from build123d import *

# Parameters (mm, degrees)
SKETCH1_R                = 10
BOSS_EXTRUDE1_DEPTH      = 50
EXTRUDE_THIN1_START      = -15
SKETCH2_R                = 11
SKETCH2_R_2              = 10
EXTRUDE_THIN1_DEPTH      = 15
SKETCH3_R                = 5
BOSS_EXTRUDE2_DEPTH      = 66
CUT_EXTRUDE3_DEPTH       = 118.038455219
CUT_EXTRUDE3_DEPTH_BACK  = 118.038455219
SKETCH4_R                = 2
EXTRUDE_THIN2_DEPTH      = 12
EXTRUDE_THIN2_DEPTH_BACK = 12
SKETCH5_R                = 11
SKETCH5_R_2              = 10
CUT_EXTRUDE4_DEPTH       = 118.038455318
CUT_EXTRUDE4_DEPTH_BACK  = 118.038455318
SKETCH7_R                = 2


with BuildPart() as part:
    # Sketch1 → Boss-Extrude1 (new body)
    with BuildSketch(Plane.XY):
        Circle(SKETCH1_R)
    extrude(amount=-BOSS_EXTRUDE1_DEPTH)

    # Sketch2 → Extrude-Thin1 (add)
    with BuildSketch(Plane(origin=(0, 0, -50), x_dir=(-1, 0, 0), z_dir=(0, 0, -1)).offset(EXTRUDE_THIN1_START)):
        Circle(SKETCH2_R)
        Circle(SKETCH2_R_2, mode=Mode.SUBTRACT)
    extrude(amount=EXTRUDE_THIN1_DEPTH)

    # Sketch3 → Boss-Extrude2 (add)
    with BuildSketch(Plane(origin=(0, 0, -50), x_dir=(-1, 0, 0), z_dir=(0, 0, -1))):
        Circle(SKETCH3_R)
    extrude(amount=BOSS_EXTRUDE2_DEPTH)

    # Sketch4 → Cut-Extrude3 (cut, two sides: drawn at the far end of the back side and taken through both)
    with BuildSketch(Plane(origin=(0, 0, 0), x_dir=(0, 0, -1), z_dir=(1, 0, 0)).offset(-CUT_EXTRUDE3_DEPTH_BACK)):
        with Locations((110.360244091, 0)):
            Circle(SKETCH4_R)
    extrude(amount=CUT_EXTRUDE3_DEPTH + CUT_EXTRUDE3_DEPTH_BACK, mode=Mode.SUBTRACT)

    # Sketch5 → Extrude-Thin2 (add, two sides: drawn at the far end of the back side and taken through both)
    with BuildSketch(Plane.XY.offset(-EXTRUDE_THIN2_DEPTH_BACK)):
        Circle(SKETCH5_R)
        Circle(SKETCH5_R_2, mode=Mode.SUBTRACT)
    extrude(amount=EXTRUDE_THIN2_DEPTH + EXTRUDE_THIN2_DEPTH_BACK)

    # Sketch7 → Cut-Extrude4 (cut, two sides: drawn at the far end of the back side and taken through both)
    with BuildSketch(Plane(origin=(0, 0, 0), x_dir=(0, 0, -1), z_dir=(1, 0, 0)).offset(-CUT_EXTRUDE4_DEPTH_BACK)):
        with Locations((-5.38623627, 0)):
            Circle(SKETCH7_R)
    extrude(amount=CUT_EXTRUDE4_DEPTH + CUT_EXTRUDE4_DEPTH_BACK, mode=Mode.SUBTRACT)


solid = part.part
Work out the finished part from the listing and answer in its coordinate system (mm). A direction names the side the tool comes from. Coordinates: 2 decimals unless noted, no trailing zeros. Write each loop counter-clockwise with the first axis right and the second up, starting at its lowest first coordinate (ties: lowest second). Pieces come first, ordered by that corner, then holes. Notation, with made-up numbers: M 48,42.5 L 85,42.5 A21 cw 85,65.5 Z; hole C 74.25,69.25 d5. An arc over 180 degrees is marked long. Use one line per item in the form item = value. Start each with the question number.
1. The part is cut by section C-C (z = -21). Give the vertices of the cut face in (x, y), plus the area to 3 significant figures.
2. The part is cut by section A-A (y = 0). Give the number of separate pieces and of enclosed holes in the cut face, plus the area to 3 significant figures.
3. Straight lines are drawn through the part: probe 1 along Z at (x, y) = (-0.5, 0); probe 2 along Y at (x, z) = (0, 6.5); probe 3 along Z at (x, y) = (3, 7.75). For each, find the intervals that lie inside material, in ascending order. Write a range as from..to.
4. The part is cut by section D-D (x = -8.5). Give the vertices of the cut face in (y, z).
5. The mould has two halves that part along Y. Classify faces 1 (the face through (0, 0, -116)), 2 (the face through (0, 0, 0)), 3 (the face through (-4.619, -1.915, -82.538)): released by +Y, released by -Y, zero draft, split by the parting line, or undercut.
6. The part is cut by section B-B (x = 0). Give the vertices of the cut face in (y, z).
7. A tool of negligible diameter and unlimited length cuts with its end or side. For faces 4 (the face through (9.54, 3, 5.92)), 5 (the face through (-2, -5, -50)), 6 (the face through (-2, -10, -35)), 7 (the face through (10.391, -1.774, 4.463)), from which of +Z, -Z, +X, -X, +Y, -Y can it reach the whole face along a straight path? Write none if from no direction.
8. Each of these flat-tipped pins is pushed along its axis until it touches: P1, Ø6, axis at x = -2, z = -93.5, coming from the +Y side; P2, Ø2.5, axis at y = 0, z = 5.39, coming from the +X side; P3, Ø12, axis at x = 3, z = -23, coming from the +Y side; P4, Ø2, axis at x = 5, z = -31.5, coming from the +Y side. Where does it stop, or does it pass through?
Evaluation:
q1.outline = C 0,0 d20
q1.area = 314 mm^2
q2.separate_pieces = 4
q2.enclosed_holes = 0
q2.area = 1,690 mm^2
q3.probe_1 = -116..-112.36, -108.36..0
q3.probe_2 = -11..-10, 10..11
q3.probe_3 = -50..0
q4.outline = M -6.98,-50 L 6.98,-50 L 6.98,-35 L 5.27,-35 L 5.27,-12 L 6.98,-12 L 6.98,12 L 5.27,12 L 5.27,0 L -5.27,0 L -5.27,12 L -6.98,12 L -6.98,-12 L -5.27,-12 L -5.27,-35 L -6.98,-35 Z
q5.face_1 = zero draft
q5.face_2 = undercut
q5.face_3 = split by the parting line
q6.outline = M -11,-50 L -5,-50 L -5,-116 L 5,-116 L 5,-50 L 11,-50 L 11,-35 L 10,-35 L 10,-12 L 11,-12 L 11,12 L 10,12 L 10,0 L -10,0 L -10,12 L -11,12 L -11,-12 L -10,-12 L -10,-35 L -11,-35 Z; hole C 0,-110.36 d4
q7.face_4 = +Z
q7.face_5 = -Z
q7.face_6 = none
q7.face_7 = +X, -X
q8.P1 = 5
q8.P2 = through
q8.P3 = 10
q8.P4 = 9.17
